Geometry: see drawing. Coordinates: mm, zero at the bounding-box minimum. A direction names the side the tool comes from. Round coordinates to 2 decimals unless told otherwise and drop trailing zeros. Loops run counter-clockwise (first coordinate to the right, second up) from the corner with the lowest first, then second, coordinate; pieces in that order, holes last. Notation, with made-up numbers: M -33,17.5 L 23,17.5 A25 ccw 23,53.5 Z; hole C 80.5,-22.75 d7. An arc over 180 degrees is marked long. Answer as a JSON object with one key per item and string values.
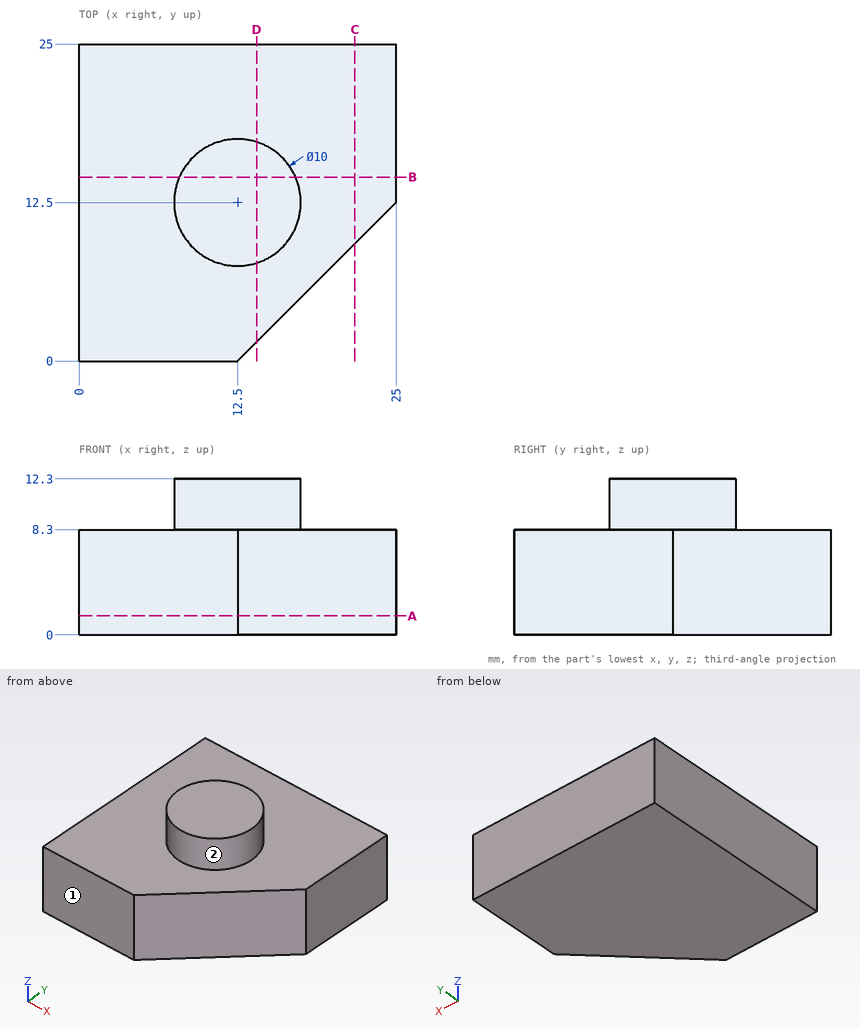
1) Section query B-B (y = 14.5). Return the cut outline in (x, z).
Results:
{"outline": "M 0,0 L 25,0 L 25,8.3 L 17.08,8.3 L 17.08,12.3 L 7.92,12.3 L 7.92,8.3 L 0,8.3 Z"}
2) Section query C-C (x = 21.75). Return the cut outline in (y, z), and give its area (3 significant figures).
Results:
{"outline": "M 9.25,0 L 25,0 L 25,8.3 L 9.25,8.3 Z", "area": "131 mm2"}
3) Ray query, line 1 (Z direction, x = 8, y = 5.75); line 2 (Y direction, x = 15.25, z = 5.75); line 3 (X direction, y = 8.5, z = 7.25). Return the intervals inside material, ascending.
Results:
{"line 1": "0 to 8.3", "line 2": "2.75 to 25", "line 3": "0 to 21"}
4) Section query D-D (x = 14). Return the cut outline in (y, z).
Results:
{"outline": "M 1.5,0 L 25,0 L 25,8.3 L 17.27,8.3 L 17.27,12.3 L 7.73,12.3 L 7.73,8.3 L 1.5,8.3 Z"}
5) Reachability of the marked faces 1 and 2 from +Z, -Z, +X, -X, +Y, -Y: full face, straight path, thin tool, end or side. Return the list, or none.
Results:
{"face 1": "+Z, -Z, +X, -X, -Y", "face 2": "+Z"}
6) Section query A-A (z = 1.5). Return the cut outline in (x, y).
Results:
{"outline": "M 0,0 L 12.5,0 L 25,12.5 L 25,25 L 0,25 Z"}
7) Pin query (flat end, axial travel): P1, Ø3, axis at y = 9, z = 7, coming from the +X side; P2, Ø1, axis at x = 19, y = 4.5, coming from the -Z side. Return the tip coordinate at first contact, or that it passes through.
Results:
{"P1": "x = 23", "P2": "through"}
